from build123d import *

# Parameters (mm, degrees)
CROQUIS1_R              = 2.5
SALIENTE_EXTRUIR2_DEPTH = 22.5


with BuildPart() as part:
    # Croquis1 → Saliente-Extruir2 (new body)
    with BuildSketch(Plane.XY):
        with BuildLine():
            Line((0, 0), (0, 49.8562756))
            ThreePointArc((0, 49.8562756), (-0.768605016, 57.248148258), (-2, 49.919150955))
            Line((-2, 49.919150955), (-2, 7.5))
            Line((-2, 7.5), (0, 0))
        make_face()
        with Locations((-0.886438093, 53.5)):
            Circle(CROQUIS1_R, mode=Mode.SUBTRACT)
    extrude(amount=SALIENTE_EXTRUIR2_DEPTH)


solid = part.part
The model under review builds one solid part; all positions refer to its coordinate system, in mm. A direction names the side the tool comes from. Give positions to 0.01 mm unless a question says otherwise; leave off trailing zeros. Write each loop counter-clockwise with the first axis right and the second up, starting at its lowest first coordinate (ties: lowest second). Pieces come first, ordered by that corner, then holes.
1. Add section D-D, the plane y = 8. Write out the cut boundary in (x, z).
2. Add section A-A, the plane z = 7.75. Write out the cut boundary in (x, y), plus the area to 3 significant figures.
3. Add section B-B, the plane y = 53.5. Write out the cut boundary in (x, z).
4. Add section C-C, the plane x = -0.75. Write out the cut boundary in (y, z).
5. Draft analysis for pull direction X (two halves, no side actions). For faces 1 (the cylindrical face through (-1.43, 51.06, 11.09)), 2 (the flat face through (-2, 29, 11)), 3 (the cylindrical face through (-0.62, 57.24, 11.09)), state which applies: +X half, -X half, draft (parallel to the pull), parting line (faces both ways), or undercut.
6. Wall thickness on L1, parallel to X at y = 35.5, z = 11.5; L2, parallel to Y at x = 1, z = 13.75; L3, parallel to Y at x = 0.75, z = 14.25: over which ranges is each line inside the solid? List them lowest first.
7. Tool access review of faces 4 (the flat face through (-1, 33, 22.5)), 5 (the flat face through (0, 25, 11)): name each direction out of +Z, -Z, +X, -X, +Y, -Y from which nothing blocks a thin tool from reaching the whole face with its end or side.
8. For P1, Ø1.5, axis at x = 2, z = 7, coming from the -Y side; P2, Ø4, axis at x = -0.89, y = 53.5, coming from the +Z side; P3, Ø5, axis at y = 22, z = 5.5, coming from the +X side, all flat-tipped, find the tip position at first contact; note any pin that passes through.
Worked answers:
1. outline: (-2, 0) - (0, 0) - (0, 22.5) - (-2, 22.5) - close
2. outline: (-2, 7.5) - (0, 0) - (0, 49.86) arc R3.75 ccw (long way) to (-2, 49.92) - close; hole circle Ø5 at (-0.89, 53.5)
2. area: 117 mm2
3. outline: (-4.64, 0) - (-3.39, 0) - (-3.39, 22.5) - (-4.64, 22.5) - close; (1.61, 0) - (2.86, 0) - (2.86, 22.5) - (1.61, 22.5) - close
4. outline: (2.81, 0) - (51, 0) - (51, 22.5) - (2.81, 22.5) - close; (56, 0) - (57.25, 0) - (57.25, 22.5) - (56, 22.5) - close
5. face 1: undercut
5. face 2: -X half
5. face 3: parting line
6. L1: x = -2 to 0
6. L2: y = 50.26 to 51.86, 55.14 to 56.74
6. L3: y = 50.13 to 51.61, 55.39 to 56.87
7. face 4: +Z, +X, -X, +Y, -Y
7. face 5: +Z, -Z, +X, -Y
8. P1: stops at y = 50.42
8. P2: passes through
8. P3: stops at x = 0
